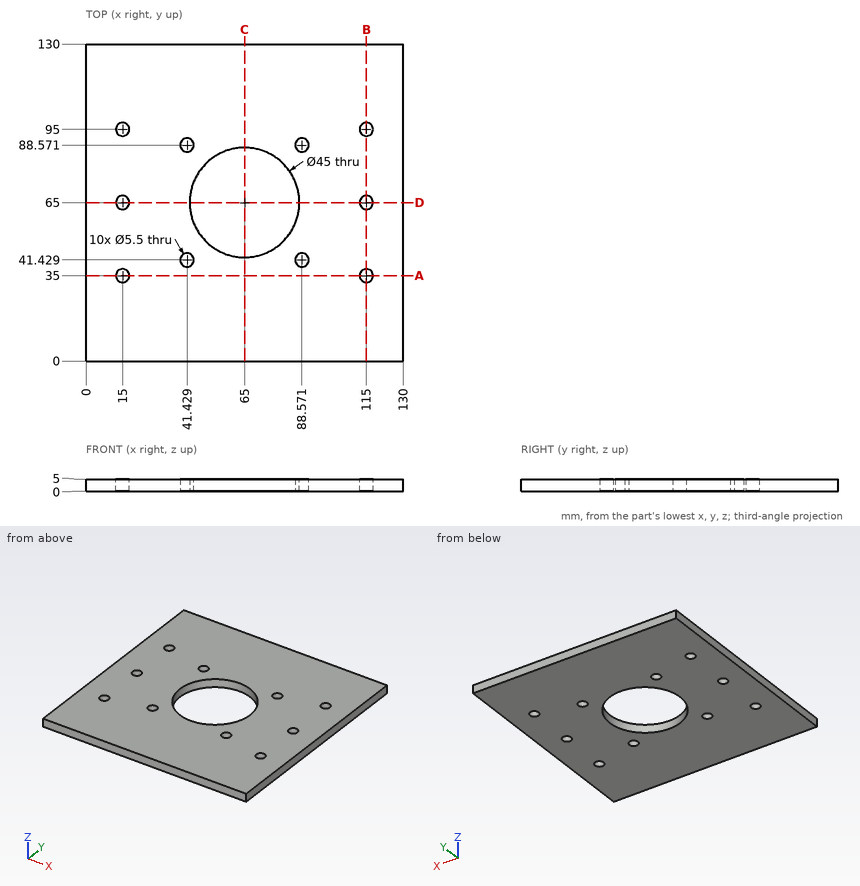
Geometry check sheet. Reference: drawing and pictorial views, mm from the part's lowest x, y, z. Round coordinates to 2 decimals unless told otherwise and drop trailing zeros. Loops run counter-clockwise (first coordinate to the right, second up) from the corner with the lowest first, then second, coordinate; pieces in that order, holes last. Notation, with made-up numbers: (40.25, 78.25) -> (81.25, 78.25) arc R29 cw to (81.25, 105.25) -> close; hole circle Ø2 at (18.25, 6.5). An arc over 180 degrees is marked (long way). Use a Markdown table: item, result.
(1) Sectioned sample at D-D (y = 65). Enter the section's corners in (x, z).
Calculated:
| item | result |
|---|---|
| outline | (0, 0) -> (12.25, 0) -> (12.25, 5) -> (0, 5) -> close; (17.75, 0) -> (42.5, 0) -> (42.5, 5) -> (17.75, 5) -> close; (87.5, 0) -> (112.25, 0) -> (112.25, 5) -> (87.5, 5) -> close; (117.75, 0) -> (130, 0) -> (130, 5) -> (117.75, 5) -> close |
(2) Go/stop test with a flat-tipped pin: P1, Ø7, axis at x = 115, y = 35, coming from the -Z side. Record where the tip stops, or that it passes through.
Calculated:
| item | result |
|---|---|
| P1 | z = 0 |
(3) Sectioned sample at C-C (x = 65). Enter the section's corners in (y, z), then the cut area to 3 significant figures.
Calculated:
| item | result |
|---|---|
| outline | (0, 0) -> (42.5, 0) -> (42.5, 5) -> (0, 5) -> close; (87.5, 0) -> (130, 0) -> (130, 5) -> (87.5, 5) -> close |
| area | 425 mm² |
(4) Sectioned sample at B-B (x = 115). Enter the section's corners in (y, z).
Calculated:
| item | result |
|---|---|
| outline | (0, 0) -> (32.25, 0) -> (32.25, 5) -> (0, 5) -> close; (37.75, 0) -> (62.25, 0) -> (62.25, 5) -> (37.75, 5) -> close; (67.75, 0) -> (92.25, 0) -> (92.25, 5) -> (67.75, 5) -> close; (97.75, 0) -> (130, 0) -> (130, 5) -> (97.75, 5) -> close |
(5) Sectioned sample at A-A (y = 35). Enter the section's corners in (x, z).
Calculated:
| item | result |
|---|---|
| outline | (0, 0) -> (12.25, 0) -> (12.25, 5) -> (0, 5) -> close; (17.75, 0) -> (112.25, 0) -> (112.25, 5) -> (17.75, 5) -> close; (117.75, 0) -> (130, 0) -> (130, 5) -> (117.75, 5) -> close |
(6) Scan lines: probe 1 along Y at (x, z) = (15, 1.75); probe 2 along X at (y, z) = (41, 2) (1 decimal); probe 3 along Y at (x, z) = (65, 3.8). Record each from-to range of solid material in increasing order.
Calculated:
| item | result |
|---|---|
| probe 1 | 0 to 32.25, 37.75 to 62.25, 67.75 to 92.25, 97.75 to 130 |
| probe 2 | 0 to 38.7, 44.1 to 85.9, 91.3 to 130 |
| probe 3 | 0 to 42.5, 87.5 to 130 |
